Read the model definition and answer for the solid it produces. Units are mm, in the model's axes. A direction names the side the tool comes from. Give positions to 0.01 mm unless a question says otherwise; leave off trailing zeros. Write each loop counter-clockwise with the first axis right and the second up, starting at its lowest first coordinate (ties: lowest second). Pieces come first, ordered by that corner, then holes.
```python
from build123d import *

# Parameters (mm, degrees)
F0_W     = 8
F0_H     = 3.175
F1_DEPTH = 3.175


# Not quite as in the source:
# - a length typed as a fraction of an inch, garbled in the dataset ("3 / 203.2 mm" for 3/8 in), is restored
# - a feature names something its author has since deleted; it is built from what else it names


with BuildPart() as f1:
    # F0 (on Top) → F1 (new body)
    with BuildSketch(Plane.XY):
        Polygon((-19.325, 11.15), (19.325, 11.15), (19.325, 16.15), (22.5, 16.15), (22.5, 22.5), (-22.5, 22.5), (-22.5, 16.15), (-19.325, 16.15), align=None)
        Polygon((-19.325, -11.15), (19.325, -11.15), (19.325, -6.15), (22.5, -6.15), (22.5, 6.15), (19.325, 6.15), (19.325, 11.15), (-19.325, 11.15), (-19.325, 6.15), (-22.5, 6.15), (-22.5, -6.15), (-19.325, -6.15), align=None)
        with BuildLine():
            ThreePointArc((-8.9444444444, -0.9984555975), (-10, 0), (-8.9444444444, 0.9984555975))
            ThreePointArc((-8.9444444444, 0.9984555975), (-6.000579123, 6.7076859042), (0, 9))
            ThreePointArc((0, 9), (6.000579123, 6.7076859042), (8.9444444444, 0.9984555975))
            ThreePointArc((8.9444444444, 0.9984555975), (9.6871842709, 0.7264831573), (10, 0))
            ThreePointArc((10, 0), (9.6871842709, -0.7264831573), (8.9444444444, -0.9984555975))
            ThreePointArc((8.9444444444, -0.9984555975), (6.000579123, -6.7076859042), (0, -9))
            ThreePointArc((0, -9), (-6.000579123, -6.7076859042), (-8.9444444444, -0.9984555975))
        make_face(mode=Mode.SUBTRACT)
        Polygon((-22.5, -22.5), (22.5, -22.5), (22.5, -16.15), (19.325, -16.15), (19.325, -11.15), (-19.325, -11.15), (-19.325, -16.15), (-22.5, -16.15), align=None)
        with BuildLine():
            ThreePointArc((-0.9980449639, 7.9375), (-5.9993482859, 5.2922415047), (-8, 0))
            ThreePointArc((-8, 0), (-5.9993482859, -5.2922415047), (-0.9980449639, -7.9375))
            ThreePointArc((-0.9980449639, -7.9375), (0, -7), (0.9980449639, -7.9375))
            ThreePointArc((0.9980449639, -7.9375), (5.9993482859, -5.2922415047), (8, 0))
            ThreePointArc((8, 0), (5.9993482859, 5.2922415047), (0.9980449639, 7.9375))
            ThreePointArc((0.9980449639, 7.9375), (0, 7), (-0.9980449639, 7.9375))
        make_face()
        Rectangle(F0_W, F0_H, mode=Mode.SUBTRACT)
        with BuildLine():
            ThreePointArc((-8.9444444444, 0.9984555975), (-8.2735168427, 0.6871842709), (-8, 0))
            ThreePointArc((-8, 0), (-5.9993482859, 5.2922415047), (-0.9980449639, 7.9375))
            ThreePointArc((-0.9980449639, 7.9375), (-0.7288689869, 8.6846531969), (0, 9))
            ThreePointArc((0, 9), (-6.000579123, 6.7076859042), (-8.9444444444, 0.9984555975))
        make_face()
        with BuildLine():
            ThreePointArc((8.9444444444, 0.9984555975), (6.000579123, 6.7076859042), (0, 9))
            ThreePointArc((0, 9), (0.7071067812, 8.7071067812), (1, 8))
            ThreePointArc((1, 8), (0.9995111215, 7.9687347151), (0.9980449639, 7.9375))
            ThreePointArc((0.9980449639, 7.9375), (5.9993482859, 5.2922415047), (8, 0))
            ThreePointArc((8, 0), (8.2735168427, 0.6871842709), (8.9444444444, 0.9984555975))
        make_face()
        with BuildLine():
            ThreePointArc((1, -8), (0.7071067812, -8.7071067812), (0, -9))
            ThreePointArc((0, -9), (6.000579123, -6.7076859042), (8.9444444444, -0.9984555975))
            ThreePointArc((8.9444444444, -0.9984555975), (8.2735168427, -0.6871842709), (8, 0))
            ThreePointArc((8, 0), (5.9993482859, -5.2922415047), (0.9980449639, -7.9375))
            ThreePointArc((0.9980449639, -7.9375), (0.9995111215, -7.9687347151), (1, -8))
        make_face()
        with BuildLine():
            ThreePointArc((-0.9980449639, -7.9375), (-5.9993482859, -5.2922415047), (-8, 0))
            ThreePointArc((-8, 0), (-8.2735168427, -0.6871842709), (-8.9444444444, -0.9984555975))
            ThreePointArc((-8.9444444444, -0.9984555975), (-6.000579123, -6.7076859042), (0, -9))
            ThreePointArc((0, -9), (-0.7288689869, -8.6846531969), (-0.9980449639, -7.9375))
        make_face()
    extrude(amount=F1_DEPTH)


solid = f1.part
```
Item 1: Section B-B (z = 2.5) is taken. Give the number of separate pieces and of enclosed holes in the cut face, and give its area (3 significant figures).
Result set:
separate pieces: 1
enclosed holes: 5
area: 1,860 mm2
Item 2: Which of the six approach directions +Z, -Z, +X, -X, +Y, -Y give full straight-line access (tool end or side, diameter ignored) to faces 1 (the flat face through (-21, -6.15, 2)), 2 (the flat face through (0, -1.588, 2)), 3 (the flat face through (21, -6.15, 2))?
Result set:
face 1: +Z, -Z, -X
face 2: +Z, -Z
face 3: +Z, -Z, +X
Item 3: Determine the mould class of faces 4 (the flat face through (22.5, 0, 2)), 5 (the flat face through (0, 1.588, 2)), 6 (the flat face through (21, 6.15, 2)) for opening direction X: pulls with the +X half, pulls with the -X half, needs draft (parallel to the pull), parting line crosses it, or undercut.
Result set:
face 4: pulls with the +X half
face 5: undercut
face 6: needs draft
Item 4: Find the intervals of material crossed by line 1 along Y through (x, z) = (-3.5, 1.9); line 2 along X through (y, z) = (14, 2.4) (3 decimals), in increasing order.
Result set:
line 1: y = -22.5 to -1.59, 1.59 to 22.5
line 2: x = -19.325 to 19.325
Item 5: Each of these flat-tipped pins is pushed along its axis until it touches: pin 1 Ø1.6 at (y, z) = (10, 2) entering from +X (3 decimals); pin 2 Ø1.6 at (y, z) = (-10.5, 1.5) entering from -X (3 decimals). Where does it stop, or does it pass through?
Result set:
pin 1: stops at x = 19.325
pin 2: stops at x = -19.325
Item 6: Section A-A (y = -10) is taken. Write down the section's boundary in (x, z) (3 decimals), and give its area (3 significant figures).
Result set:
outline: (-19.325, 0) - (19.325, 0) - (19.325, 3.175) - (-19.325, 3.175) - close
area: 123 mm2
